from build123d import *

# Parameters (mm, degrees)
BOSS_EXTRUDE1_DEPTH       = 76.2
TAP_DRILL_FOR_8_36_TAP1_D = 3.4544
TAP_DRILL_FOR_8_36_TAP2_D = 3.4544


with BuildPart() as part:
    # Sketch1 → Boss-Extrude1 (new body)
    with BuildSketch(Plane.XY):
        Polygon((0, 0), (0, 28.575), (-79.375, 28.575), (-79.375, 25.4), (-3.175, 25.4), (-3.175, 0), align=None)
    extrude(amount=BOSS_EXTRUDE1_DEPTH)

    # Tap Drill for #8-36 Tap1 (through all)
    with Locations(Plane.ZY.offset(3.175)):
        with Locations((38.1, 6.6), (38.1, 19.3)):
            Hole(TAP_DRILL_FOR_8_36_TAP1_D / 2)

    # Tap Drill for #8-36 Tap2 (through all)
    with Locations(Plane(origin=(0, 25.4, 0), x_dir=(-1, 0, 0), z_dir=(0, -1, 0))):
        with Locations((60.325, -63.5), (22.225, -63.5), (60.325, -13.711593905), (22.225, -13.711593905)):
            Hole(TAP_DRILL_FOR_8_36_TAP2_D / 2)


solid = part.part
Geometry: final body of the model. Coordinates: model frame, mm. A direction names the side the tool comes from. Round coordinates to 2 decimals unless told otherwise and drop trailing zeros. Loops run counter-clockwise (first coordinate to the right, second up) from the corner with the lowest first, then second, coordinate; pieces in that order, holes last.
Q1. Access query for faces 1 (the flat face through (-31, 27, 76.2)), 2 (the flat face through (-3.175, 13, 38)). Directions: +Z, -Z, +X, -X, +Y, -Y. A direction counts if a zero-diameter tool reaches every point of the face in a straight line with its end or side. Return the directions, or none.
Q2. Material intervals for L1, parallel to Y at x = -1, z = 38 (3 decimals); L2, parallel to Y at x = -52, z = 12.5 (3 decimals); L3, parallel to X at y = 9.5, z = 52 (3 decimals), sorted ascending.
Q3. Section C-C on z = 21. Return loops of the section in (x, y) (3 decimals).
Q4. Section A-A on z = 63.5. Return loops of the section in (x, y) (3 decimals), plus the area to 3 significant figures.
Q5. Section B-B on y = 19.3. Return loops of the section in (x, z) (3 decimals).
Q6. Pull-direction query (X, two-part tool) for faces 3 (the flat face through (-31, 27, 0)), 4 (the flat face through (0, 14, 38)), 5 (the cylindrical face through (-21.3, 27.01, 62.04)); classes: released by +X, released by -X, zero draft, split by the parting line, or undercut.
Q7. Pin query (flat end, axial travel): P1, Ø12.5, axis at y = 17.5, z = 39.5, coming from the -X side (3 decimals); P2, Ø3, axis at x = -60.32, z = 13.71, coming from the -Y side; P3, Ø23, axis at x = -32, z = 46, coming from the -Y side. Return the tip coordinate at first contact, or that it passes through.
Q8. Section D-D on x = -70.5. Return loops of the section in (y, z) (3 decimals).
Evaluation:
1. face 1: +Z, +X, -X, +Y, -Y
1. face 2: +Z, -Z, -X, -Y
2. L1: y = 0 to 4.876, 8.324 to 17.576, 21.024 to 28.575
2. L2: y = 25.4 to 28.575
2. L3: x = -3.175 to 0
3. outline: (-79.375, 25.4) - (-3.175, 25.4) - (-3.175, 0) - (0, 0) - (0, 28.575) - (-79.375, 28.575) - close
4. outline: (-79.375, 25.4) - (-62.052, 25.4) - (-62.052, 28.575) - (-79.375, 28.575) - close; (-58.598, 25.4) - (-23.952, 25.4) - (-23.952, 28.575) - (-58.598, 28.575) - close; (-20.498, 25.4) - (-3.175, 25.4) - (-3.175, 0) - (0, 0) - (0, 28.575) - (-20.498, 28.575) - close
4. area: 311 mm2
5. outline: (-3.175, 0) - (0, 0) - (0, 36.373) - (-3.175, 36.373) - close; (-3.175, 39.827) - (0, 39.827) - (0, 76.2) - (-3.175, 76.2) - close
6. face 3: zero draft
6. face 4: released by +X
6. face 5: undercut
7. P1: stops at x = -3.175
7. P2: passes through
7. P3: stops at y = 25.4
8. outline: (25.4, 0) - (28.575, 0) - (28.575, 76.2) - (25.4, 76.2) - close
